Check sheet for the modelled part. Datum: model origin and axes. Units: mm. A direction names the side the tool comes from. Round coordinates to 2 decimals unless told otherwise and drop trailing zeros. Write each loop counter-clockwise with the first axis right and the second up, starting at its lowest first coordinate (ties: lowest second). Pieces come first, ordered by that corner, then holes. Notation, with made-up numbers: (76.25, -34) -> (110.25, -34) arc R7 cw to (110.25, -27) -> close; hole circle Ø5 at (-10, 66.5). An arc over 180 degrees is marked (long way). One line per item, written item: value.
from build123d import *

# Parameters (mm, degrees)
BOSS_EXTRUDE1_DEPTH  = 3
M3_CLEARANCE_HOLE1_D = 3.4
M4_CLEARANCE_HOLE1_D = 4.5
FILLET1_R            = 3


with BuildPart() as part:
    # Sketch1 → Boss-Extrude1 (new body)
    with BuildSketch(Plane.XY):
        with BuildLine():
            Line((50.773782993, 15), (50.773782993, 41.5958))
            ThreePointArc((50.773782993, 41.5958), (59.386891497, 50.208908503), (68, 41.5958))
            Line((68, 41.5958), (68, 15))
            Line((68, 15), (78, 15))
            Line((78, 15), (78, -15))
            Line((78, -15), (40.773782993, -15))
            Line((40.773782993, -15), (40.773782993, 15))
            Line((40.773782993, 15), (50.773782993, 15))
        make_face()
    extrude(amount=BOSS_EXTRUDE1_DEPTH)

    # M3 Clearance Hole1 (through all)
    with Locations(Plane.XY.offset(3)):
        with Locations((59.40350934, 41.5958)):
            Hole(M3_CLEARANCE_HOLE1_D / 2)

    # M4 Clearance Hole1 (through all)
    with Locations(Plane.XY.offset(3)):
        with Locations((46.773782993, 0), (72, 0), (59.177120078, 0)):
            Hole(M4_CLEARANCE_HOLE1_D / 2)

    # Fillet1
    fillet1_edges = [part.edges().sort_by_distance(p)[0] for p in [
        (78, -15, 1.5),
        (40.773782993, -15, 1.5),
        (40.773782993, 15, 1.5),
        (78, 15, 1.5),
    ]]
    fillet(fillet1_edges, radius=FILLET1_R)


solid = part.part
Item 1: Sectioned sample at A-A on x = 72. Enter the section's corners in (y, z).
Answer:
outline: (-15, 0) -> (-2.25, 0) -> (-2.25, 3) -> (-15, 3) -> close; (2.25, 0) -> (15, 0) -> (15, 3) -> (2.25, 3) -> close
Item 2: Sectioned sample at C-C on z = 1.9. Enter the section's corners in (x, y), and give its area (3 significant figures).
Answer:
outline: (40.77, -12) arc R3 ccw to (43.77, -15) -> (75, -15) arc R3 ccw to (78, -12) -> (78, 12) arc R3 ccw to (75, 15) -> (68, 15) -> (68, 41.6) arc R8.61 ccw to (50.77, 41.6) -> (50.77, 15) -> (43.77, 15) arc R3 ccw to (40.77, 12) -> close; hole circle Ø4.5 at (46.77, 0); hole circle Ø4.5 at (59.18, 0); hole circle Ø3.4 at (59.4, 41.6); hole circle Ø4.5 at (72, 0)
area: 1,630 mm^2
Item 3: Thickness scan on line 1 (Y direction, x = 59, z = 1.25); line 2 (X direction, y = 2, z = 1.2); line 3 (Y direction, x = 72, z = 1.9). Record the ranges inside material, lowest first.
Answer:
line 1: y = -15 to -2.24, 2.24 to 39.94, 43.25 to 50.2
line 2: x = 40.77 to 45.74, 47.8 to 58.15, 60.21 to 70.97, 73.03 to 78
line 3: y = -15 to -2.25, 2.25 to 15
Item 4: Sectioned sample at B-B on y = 0. Enter the section's corners in (x, z), and give its area (3 significant figures).
Answer:
outline: (40.77, 0) -> (44.52, 0) -> (44.52, 3) -> (40.77, 3) -> close; (49.02, 0) -> (56.93, 0) -> (56.93, 3) -> (49.02, 3) -> close; (61.43, 0) -> (69.75, 0) -> (69.75, 3) -> (61.43, 3) -> close; (74.25, 0) -> (78, 0) -> (78, 3) -> (74.25, 3) -> close
area: 71.2 mm^2
Item 5: Depth check by flat-ended pin: P1, Ø1.5, axis at x = 73, z = 1, coming from the +Y side; P2, Ø0.9, axis at y = 35, z = 2, coming from the +X side. Enter the tip coordinate at first touch or a pass-through.
Answer:
P1: stops at y = 15
P2: stops at x = 68
Item 6: Tool access check on faces 5 (the cylindrical face through (69.92, -0.86, 1.48)), 6 (the flat face through (47, 15, 1)), 7 (the flat face through (68, 28, 1)). Record the directions out of +Z, -Z, +X, -X, +Y, -Y that give a thin tool (end or side, any length) a straight path to the whole face; none if there is none.
Answer:
face 5: +Z, -Z
face 6: +Z, -Z, -X, +Y
face 7: +Z, -Z, +X, +Y
Item 7: Mould release check, pull along Y, two halves, no side actions. Record for faces 1 (the cylindrical face through (59.62, 43.28, 1.48)), 2 (the flat face through (40.774, 0, 1)), 3 (the cylindrical face through (59.197, 50.207, 1.479)), 4 (the cylindrical face through (61.425, 0.099, 1.479)): pulls with the +Y half, pulls with the -Y half, needs draft (parallel to the pull), parting line crosses it, or undercut.
Answer:
face 1: undercut
face 2: needs draft
face 3: pulls with the +Y half
face 4: undercut
Item 8: Sectioned sample at D-D on x = 59. Enter the section's corners in (y, z), and give its area (3 significant figures).
Answer:
outline: (-15, 0) -> (-2.24, 0) -> (-2.24, 3) -> (-15, 3) -> close; (2.24, 0) -> (39.94, 0) -> (39.94, 3) -> (2.24, 3) -> close; (43.25, 0) -> (50.2, 0) -> (50.2, 3) -> (43.25, 3) -> close
area: 172 mm^2
